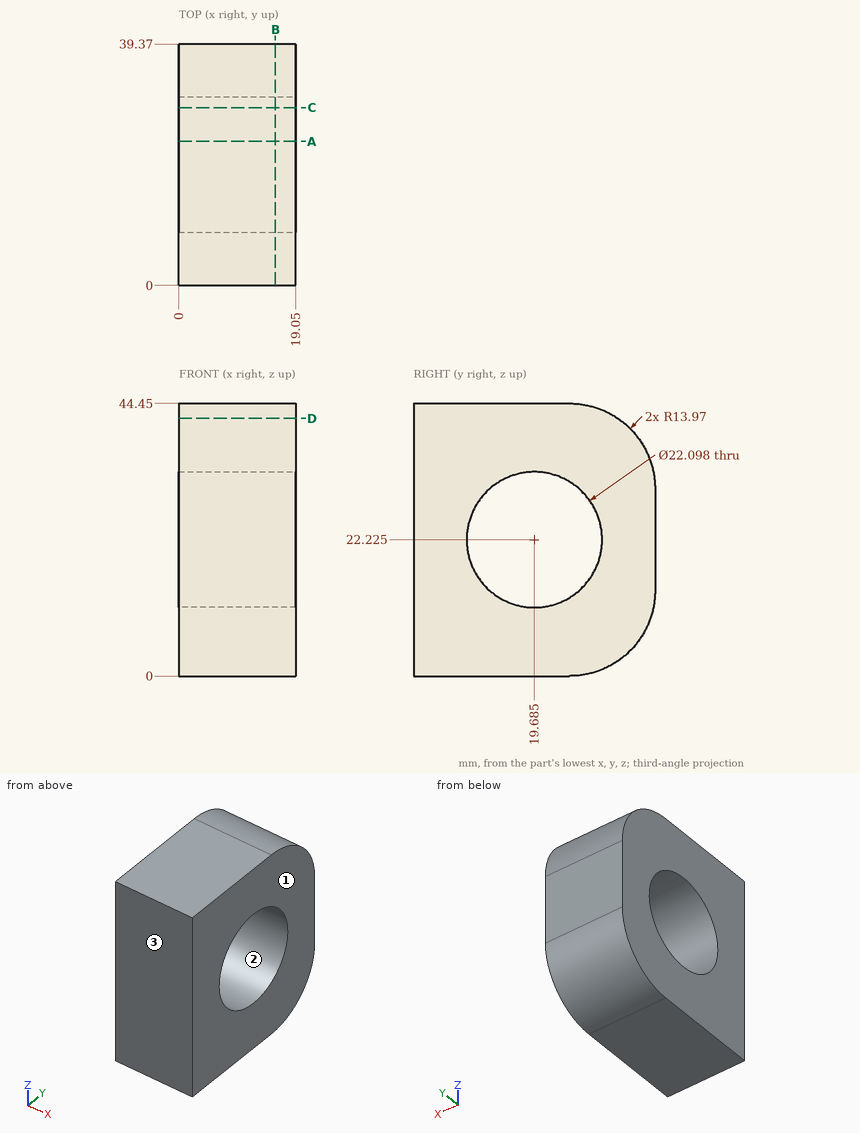
Source: three-view drawing plus pictorial views. Frame: mm from the lowest corner of the part. Coordinates: 2 decimals unless noted, no trailing zeros. Loops run counter-clockwise (first coordinate to the right, second up) from the corner with the lowest first, then second, coordinate; pieces in that order, holes last. Notation, with made-up numbers: (45.25, -8.75) - (49.25, -8.75) arc R32 ccw to (49.25, 24.25) - close; hole circle Ø6 at (46, 18.25). An arc over 180 degrees is marked (long way). One line per item, written item: value. Start each with the question number.
1. Section D-D (z = 42). Return the cut outline in (x, y), and give its area (3 significant figures).
2. Mould query, pull axis Y, two halves, no side actions, for the marked faces 1, 2 and 3. Classes: pulls with the +Y half, pulls with the -Y half, needs draft (parallel to the pull), parting line crosses it, or undercut.
3. Ray query, L1, parallel to Y at x = 18.25, z = 19; L2, parallel to Z at x = 6.5, y = 10.5; L3, parallel to Y at x = 7.25, z = 15.5. Return the intervals inside material, ascending.
4. Contact query for flat-ended pins moving along their axis: P1, Ø1.5, axis at x = 9.5, z = 40, coming from the -Y side; P2, Ø6, axis at x = 10.5, y = 32, coming from the +Z side. Output: stop coordinate, or through.
5. Section A-A (y = 23.5). Return the cut outline in (x, z).
6. Section C-C (y = 29). Return the cut outline in (x, z).
7. Section B-B (x = 15.75). Return the cut outline in (y, z) (3 decimals).
Verdict:
1. outline: (0, 0) - (19.05, 0) - (19.05, 33.3) - (0, 33.3) - close
1. area: 634 mm2
2. face 1: needs draft
2. face 2: undercut
2. face 3: pulls with the -Y half
3. L1: y = 0 to 9.12, 30.25 to 39.37
3. L2: z = 0 to 16.08, 28.37 to 44.45
3. L3: y = 0 to 10.92, 28.45 to 39.37
4. P1: stops at y = 0
4. P2: stops at z = 43.98
5. outline: (0, 0) - (19.05, 0) - (19.05, 11.86) - (0, 11.86) - close; (0, 32.59) - (19.05, 32.59) - (19.05, 44.45) - (0, 44.45) - close
6. outline: (0, 0.47) - (19.05, 0.47) - (19.05, 16.28) - (0, 16.28) - close; (0, 28.17) - (19.05, 28.17) - (19.05, 43.98) - (0, 43.98) - close
7. outline: (0, 0) - (25.4, 0) arc R13.97 ccw to (39.37, 13.97) - (39.37, 30.48) arc R13.97 ccw to (25.4, 44.45) - (0, 44.45) - close; hole circle Ø22.098 at (19.685, 22.225)
